from build123d import *

# Parameters (mm, degrees)
ESTRUSIONE_ESTRUSIONE1_DEPTH = 80
FORO_6_5_6_5_1_D             = 6.5
FORO_6_5_6_5_2_D             = 6.5
FORO_6_5_6_5_2_DEPTH         = 5
FORO_6_5_6_5_2_TIP           = 1.952797012
TAGLIO_ESTRUSIONE3_REACH     = 108.771
SCHIZZO10_R                  = 1.75
TAGLIO_ESTRUSIONE4_REACH     = 108.771
SCHIZZO11_R                  = 1.75
SMUSSO1_SIZE                 = 3
TAGLIO_ESTRUSIONE5_REACH     = 106.523
SCHIZZO12_R                  = 1.25


with BuildPart() as part:
    # Schizzo1 → Estrusione-Estrusione1 (new body)
    with BuildSketch(Plane.XY):
        Polygon((0, 0), (0, 50), (5, 50), (5, 5), (50, 5), (50, 0), align=None)
    extrude(amount=ESTRUSIONE_ESTRUSIONE1_DEPTH)

    # Foro Ø6.5 (6.5)-1 (through all)
    with Locations(Plane(origin=(0, 0, 0), x_dir=(-1, 0, 0), z_dir=(0, -1, 0))):
        with Locations((-17, -72), (-42, -72)):
            Hole(FORO_6_5_6_5_1_D / 2)

    # Foro Ø6.5 (6.5)-2
    with Locations(Plane.ZY):
        with Locations((72, 42), (72, 17)):
            Hole(FORO_6_5_6_5_2_D / 2, depth=FORO_6_5_6_5_2_DEPTH)
            with Locations((0, 0, -(FORO_6_5_6_5_2_DEPTH + FORO_6_5_6_5_2_TIP / 2))):  # 118° drill point
                Cone(0, FORO_6_5_6_5_2_D / 2, FORO_6_5_6_5_2_TIP, mode=Mode.SUBTRACT)

    # Schizzo10 → Taglio-Estrusione3 (cut, up to next)
    with BuildSketch(Plane.ZY, mode=Mode.PRIVATE) as taglio_estrusione3_sk1:
        with Locations((10, 40)):
            Circle(SCHIZZO10_R)
    taglio_estrusione3_tool1 = extrude(taglio_estrusione3_sk1.sketch, amount=-TAGLIO_ESTRUSIONE3_REACH, mode=Mode.PRIVATE) & part.part
    # Schizzo10 → Taglio-Estrusione3 (cut, up to next)
    with BuildSketch(Plane.ZY, mode=Mode.PRIVATE) as taglio_estrusione3_sk2:
        with Locations((30, 40)):
            Circle(SCHIZZO10_R)
    taglio_estrusione3_tool2 = extrude(taglio_estrusione3_sk2.sketch, amount=-TAGLIO_ESTRUSIONE3_REACH, mode=Mode.PRIVATE) & part.part
    # Schizzo10 → Taglio-Estrusione3 (cut, up to next)
    with BuildSketch(Plane.ZY, mode=Mode.PRIVATE) as taglio_estrusione3_sk3:
        with Locations((30, 20)):
            Circle(SCHIZZO10_R)
    taglio_estrusione3_tool3 = extrude(taglio_estrusione3_sk3.sketch, amount=-TAGLIO_ESTRUSIONE3_REACH, mode=Mode.PRIVATE) & part.part
    # Schizzo10 → Taglio-Estrusione3 (cut, up to next)
    with BuildSketch(Plane.ZY, mode=Mode.PRIVATE) as taglio_estrusione3_sk4:
        with Locations((10, 20)):
            Circle(SCHIZZO10_R)
    taglio_estrusione3_tool4 = extrude(taglio_estrusione3_sk4.sketch, amount=-TAGLIO_ESTRUSIONE3_REACH, mode=Mode.PRIVATE) & part.part
    add(taglio_estrusione3_tool1.solids().sort_by_distance((0, 40, 10))[0], mode=Mode.SUBTRACT)
    add(taglio_estrusione3_tool2.solids().sort_by_distance((0, 40, 30))[0], mode=Mode.SUBTRACT)
    add(taglio_estrusione3_tool3.solids().sort_by_distance((0, 20, 30))[0], mode=Mode.SUBTRACT)
    add(taglio_estrusione3_tool4.solids().sort_by_distance((0, 20, 10))[0], mode=Mode.SUBTRACT)

    # Schizzo11 → Taglio-Estrusione4 (cut, up to next)
    with BuildSketch(Plane.XZ, mode=Mode.PRIVATE) as taglio_estrusione4_sk1:
        with Locations((20, 30)):
            Circle(SCHIZZO11_R)
    taglio_estrusione4_tool1 = extrude(taglio_estrusione4_sk1.sketch, amount=-TAGLIO_ESTRUSIONE4_REACH, mode=Mode.PRIVATE) & part.part
    # Schizzo11 → Taglio-Estrusione4 (cut, up to next)
    with BuildSketch(Plane.XZ, mode=Mode.PRIVATE) as taglio_estrusione4_sk2:
        with Locations((20, 50)):
            Circle(SCHIZZO11_R)
    taglio_estrusione4_tool2 = extrude(taglio_estrusione4_sk2.sketch, amount=-TAGLIO_ESTRUSIONE4_REACH, mode=Mode.PRIVATE) & part.part
    # Schizzo11 → Taglio-Estrusione4 (cut, up to next)
    with BuildSketch(Plane.XZ, mode=Mode.PRIVATE) as taglio_estrusione4_sk3:
        with Locations((40, 50)):
            Circle(SCHIZZO11_R)
    taglio_estrusione4_tool3 = extrude(taglio_estrusione4_sk3.sketch, amount=-TAGLIO_ESTRUSIONE4_REACH, mode=Mode.PRIVATE) & part.part
    # Schizzo11 → Taglio-Estrusione4 (cut, up to next)
    with BuildSketch(Plane.XZ, mode=Mode.PRIVATE) as taglio_estrusione4_sk4:
        with Locations((40, 30)):
            Circle(SCHIZZO11_R)
    taglio_estrusione4_tool4 = extrude(taglio_estrusione4_sk4.sketch, amount=-TAGLIO_ESTRUSIONE4_REACH, mode=Mode.PRIVATE) & part.part
    add(taglio_estrusione4_tool1.solids().sort_by_distance((20, 0, 30))[0], mode=Mode.SUBTRACT)
    add(taglio_estrusione4_tool2.solids().sort_by_distance((20, 0, 50))[0], mode=Mode.SUBTRACT)
    add(taglio_estrusione4_tool3.solids().sort_by_distance((40, 0, 50))[0], mode=Mode.SUBTRACT)
    add(taglio_estrusione4_tool4.solids().sort_by_distance((40, 0, 30))[0], mode=Mode.SUBTRACT)

    # Smusso1
    smusso1_edges = [part.edges().sort_by_distance(p)[0] for p in [
        (2.5, 50, 80),
        (2.5, 50, 0),
        (50, 2.5, 80),
        (50, 2.5, 0),
    ]]
    chamfer(smusso1_edges, length=SMUSSO1_SIZE)

    # Schizzo12 → Taglio-Estrusione5 (cut, up to next)
    with BuildSketch(Plane(origin=(0, 5, 0), x_dir=(1, 0, 0), z_dir=(0, 1, 0)), mode=Mode.PRIVATE) as taglio_estrusione5_sk1:
        with Locations(Location((32, -3, 0), (0, 0, 180))):
            Circle(SCHIZZO12_R)
    taglio_estrusione5_tool1 = extrude(taglio_estrusione5_sk1.sketch, amount=-TAGLIO_ESTRUSIONE5_REACH, mode=Mode.PRIVATE) & part.part
    # Schizzo12 → Taglio-Estrusione5 (cut, up to next)
    with BuildSketch(Plane(origin=(0, 5, 0), x_dir=(1, 0, 0), z_dir=(0, 1, 0)), mode=Mode.PRIVATE) as taglio_estrusione5_sk2:
        with Locations(Location((22, -3, 0), (0, 0, 180))):
            Circle(SCHIZZO12_R)
    taglio_estrusione5_tool2 = extrude(taglio_estrusione5_sk2.sketch, amount=-TAGLIO_ESTRUSIONE5_REACH, mode=Mode.PRIVATE) & part.part
    add(taglio_estrusione5_tool1.solids().sort_by_distance((32, 5, 3))[0], mode=Mode.SUBTRACT)
    add(taglio_estrusione5_tool2.solids().sort_by_distance((22, 5, 3))[0], mode=Mode.SUBTRACT)


solid = part.part
Work out the finished part from the listing and answer in its coordinate system (mm). Give positions to 0.01 mm unless a question says otherwise; leave off trailing zeros. Loops run counter-clockwise (first coordinate to the right, second up) from the corner with the lowest first, then second, coordinate; pieces in that order, holes last. Notation, with made-up numbers: (77.25, -15) - (118.25, -15) arc R20 cw to (118.25, 9) - close; hole circle Ø5 at (-27.5, 10). An arc over 180 degrees is marked (long way). Answer in a Markdown table with one row per item. Add a question column.
Q1. Determine the mould class of faces 1 (the flat face through (0, 25, 39)), 2 (the flat face through (5, 28, 39)), 3 (the cylindrical face through (40.81, 2.46, 48.45)), 4 (the cylindrical face through (18.25, 2.46, 30.08)) for opening direction X: released by +X, released by -X, zero draft, split by the parting line, or undercut.
Q2. Consider line 1 along Z through (x, y) = (17, 2.6); line 2 along X through (y, z) = (16.5, 64.5). Determine where each line is inside the solid, lowest interval first.
Q3. The part is cut by section C-C (y = 40). Determine the outline of the cut face in (x, z), and give its area (3 significant figures).
Q4. The part is cut by section B-B (y = 17). Determine the outline of the cut face in (x, z), and give its area (4 significant figures).
Q5. Each of these flat-tipped pins is pushed along its axis until it touches: P1, Ø10, axis at y = 39.5, z = 53.5, coming from the +X side; P2, Ø8.5, axis at x = 17, z = 72, coming from the +Y side. Where does it stop, or does it pass through?
Q6. The part is cut by section A-A (x = 32). Determine the outline of the cut face in (y, z).
Q7. The part is cut by section D-D (x = 40). Determine the outline of the cut face in (y, z), and give its area (3 significant figures).
Solution:
| question | item | result |
|---|---|---|
| 1 | face 1 | released by -X |
| 1 | face 2 | released by +X |
| 1 | face 3 | undercut |
| 1 | face 4 | undercut |
| 2 | line 1 | z = 0 to 68.75, 75.25 to 80 |
| 2 | line 2 | x = 0 to 5 |
| 3 | outline | (0, 0) - (5, 0) - (5, 8.25) - (0, 8.25) - close; (0, 11.75) - (5, 11.75) - (5, 28.25) - (0, 28.25) - close; (0, 31.75) - (5, 31.75) - (5, 69.44) - (0, 69.44) - close; (0, 74.56) - (5, 74.56) - (5, 80) - (0, 80) - close |
| 3 | area | 339 mm² |
| 4 | outline | (0, 0) - (5, 0) - (5, 68.75) - (0, 68.75) - close; (0, 75.25) - (5, 75.25) - (5, 80) - (0, 80) - close |
| 4 | area | 367.5 mm² |
| 5 | P1 | stops at x = 5 |
| 5 | P2 | stops at y = 5 |
| 6 | outline | (0, 0) - (5, 0) - (5, 1.75) - (0, 1.75) - close; (0, 4.25) - (5, 4.25) - (5, 80) - (0, 80) - close |
| 7 | outline | (0, 0) - (5, 0) - (5, 28.25) - (0, 28.25) - close; (0, 31.75) - (5, 31.75) - (5, 48.25) - (0, 48.25) - close; (0, 51.75) - (5, 51.75) - (5, 69.44) - (0, 69.44) - close; (0, 74.56) - (5, 74.56) - (5, 80) - (0, 80) - close |
| 7 | area | 339 mm² |
